The listing builds one solid part. Answer for the finished solid, in the listing's coordinates (mm). Face numbers are marked on the shaded views. Round coordinates to 2 decimals unless told otherwise and drop trailing zeros. Order: outer loops, then holes, each group sorted by start corner. A loop starts at its lowest first (then second) coordinate and runs counter-clockwise, first axis right, second up. Notation, with made-up numbers: (41, 58) - (77, 58) arc R15 ccw to (77, 66) - close; hole circle Ø4 at (-8.5, 50). An arc over 180 degrees is marked (long way). One line per item, written item: value. Start each with the question number.
1. Straight lines are drawn through the part: line 1 (X direction, y = 9.25, z = 0); line 2 (X direction, y = 16, z = -2) (3 decimals); line 3 (X direction, y = -3, z = -0.5). For each, find the intervals that lie inside material, in ascending order.
2. For a pull along Y with two mould halves and no side action, classify the marked faces 1, 2, 3 and 4 as released by +Y, released by -Y, zero draft, split by the parting line, or undercut.
3. Flat-ended cylindrical pins translate along their axes: P1, Ø6, axis at x = -42.88, z = 0, coming from the -Y side; P2, Ø3, axis at x = -181, z = -5, coming from the -Y side; P3, Ø5, axis at y = -8.5, z = 11.5, coming from the -X side; P4, Ø10.5, axis at y = 0.5, z = 7, coming from the -X side. Find the tip coordinate at first contact, or state that the pin passes through.
4. Section A-A, the plane x = -187 is taken. Give the vertices of the cut face in (y, z) (1 decimal).
5. Section B-B, the plane x = -115 is taken. Give the vertices of the cut face in (y, z) (1 decimal), then the cut area to 3 significant figures.
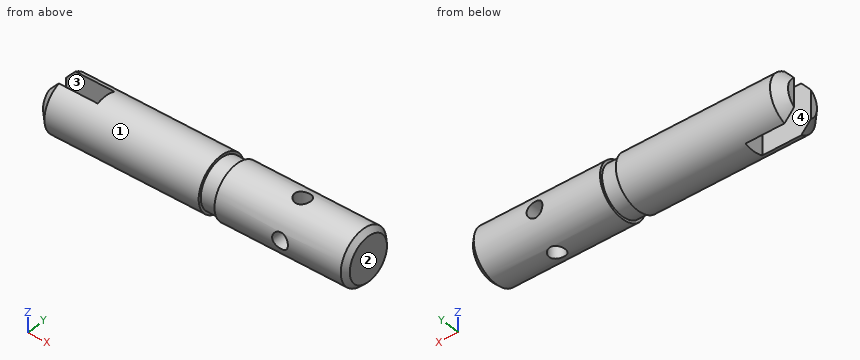
from build123d import *

# Parameters (mm, degrees)
F2_SIZE  = 6.35
F3_SIZE  = 3.175
F4_W     = 33.02
F4_H     = 12.827
F4_R     = 5.1562
F5_DEPTH = 19.05
F6_R     = 5.1562
F7_DEPTH = 19.05


with BuildPart() as f1:
    # F0 (on Top) → F1 (revolve)
    with BuildSketch(Plane.XY):
        Polygon((-203.2, 0), (0, 0), (0, 17.4625), (-85.725, 17.4625), (-85.725, 15.875), (-96.0374, 15.875), (-96.0374, 17.4625), (-203.2, 17.4625), align=None)
    revolve(axis=Axis((-82.347021, 0, 0), (1, 0, 0)))

    # F2
    f2_edges = [f1.edges().sort_by_distance(p)[0] for p in [
        (-203.2, -17.4625, 0),
    ]]
    chamfer(f2_edges, length=F2_SIZE)

    # F3
    f3_edges = [f1.edges().sort_by_distance(p)[0] for p in [
        (0, -17.4625, 0),
    ]]
    chamfer(f3_edges, length=F3_SIZE)

    # F4 (on Top) → F5 (cut, symmetric)
    with BuildSketch(Plane.XY):
        with Locations((-187.96, 0)):
            Rectangle(F4_W, F4_H)
        with Locations((-42.8752, 0)):
            Circle(F4_R)
    extrude(amount=F5_DEPTH, both=True, mode=Mode.SUBTRACT)

    # F6 (on Front) → F7 (cut, symmetric)
    with BuildSketch(Plane.XZ):
        with Locations((-42.8752, 0)):
            Circle(F6_R)
    extrude(amount=F7_DEPTH, both=True, mode=Mode.SUBTRACT)


solid = f1.part
Answer list:
1. line 1: x = -203.2 to -48.03, -37.72 to 0
1. line 2: x = -198.188 to -96.037, -85.725 to -47.628, -38.123 to -1.837
1. line 3: x = -171.45 to -48.01, -37.74 to 0
2. face 1: split by the parting line
2. face 2: zero draft
2. face 3: undercut
2. face 4: undercut
3. P1: passes through
3. P2: stops at y = -17.11
3. P3: stops at x = -202.51
3. P4: stops at x = -171.45
4. outline: (-6.4, -16.2) - (-6.4, 16.2) arc R17.5 ccw to start; (6.4, -16.2) arc R17.5 ccw to (6.4, 16.2) - close
5. outline: circle Ø34.9 at (0, 0)
5. area: 958 mm²
